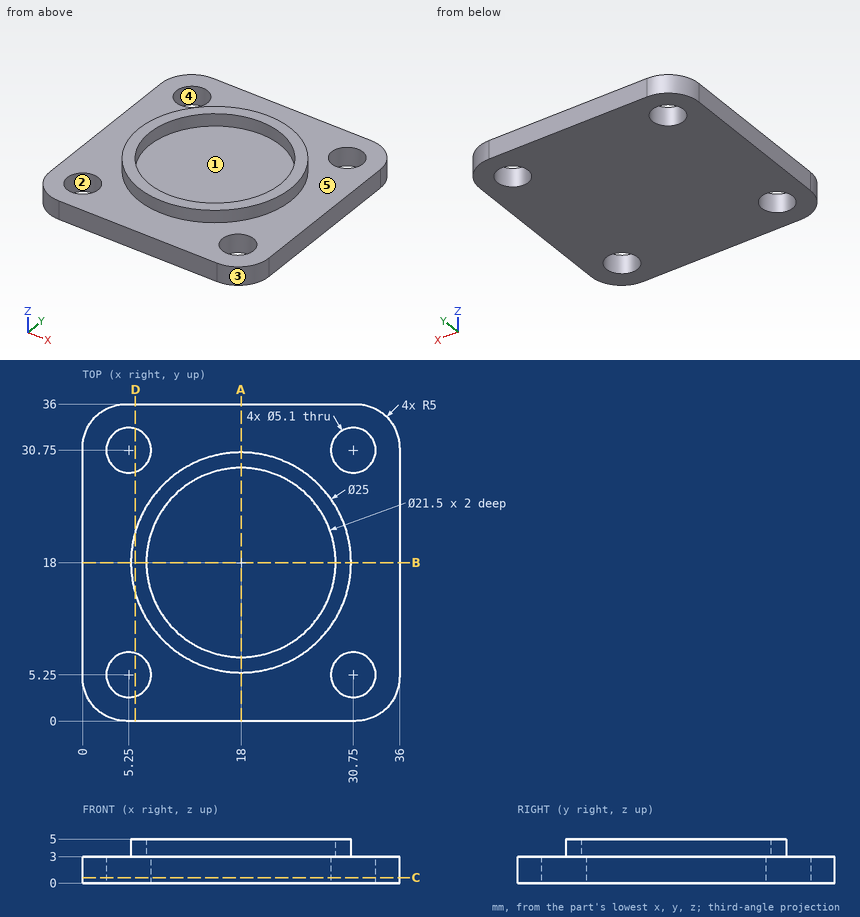
The figure shows three views and two pictorial views of one solid part (mm, origin at its lowest corner). Answer the questions. A direction names the side the tool comes from. Round coordinates to 2 decimals unless told otherwise and drop trailing zeros. Loops run counter-clockwise (first coordinate to the right, second up) from the corner with the lowest first, then second, coordinate; pieces in that order, holes last. Notation, with made-up numbers: (39, 44.25) - (81, 44.25) arc R22 cw to (81, 50.25) - close; hole circle Ø8 at (52, -30). An arc over 180 degrees is marked (long way). One line per question, with ' | ' between items. Start each with the question number.
Q1. Flat-ended cylindrical pins translate along their axes: pin 1 (6 mm diameter, centred on x = 30.75, y = 5.25, fed in from +Z); pin 2 (1 mm diameter, centred on x = 26.5, z = 4, fed in from +Y); pin 3 (3 mm diameter, centred on x = 5.25, y = 30.75, fed in from +Z). Find the tip coordinate at first contact, or state that the pin passes through.
Q2. For a pull along X with two mould halves and no side action, classify the marked faces 3, 4 and 5 as +X half, -X half, draft (parallel to the pull), parting line (faces both ways), or undercut.
Q3. Section C-C on z = 0.6 is taken. Give the vertices of the cut face in (x, y).
Q4. Section D-D on x = 6 is taken. Give the vertices of the cut face in (y, z), plus the area to 3 significant figures.
Q5. Find the intervals of material crossed by L1, parallel to Y at x = 30.75, z = 2.2; L2, parallel to Y at x = 18, z = 3.8; L3, parallel to X at y = 4.5, z = 2.2, in increasing order.
Q6. Section A-A on x = 18 is taken. Give the vertices of the cut face in (y, z).
Q7. For the marked faces 1 and 2, determine the directions among +Z, -Z, +X, -X, +Y, -Y from which every point of the face is accessible in a straight line to the end or side of a thin tool.
Established:
1) pin 1: z = 3 | pin 2: y = 27.6 | pin 3: through
2) face 3: +X half | face 4: undercut | face 5: draft
3) outline: (0, 5) arc R5 ccw to (5, 0) - (31, 0) arc R5 ccw to (36, 5) - (36, 31) arc R5 ccw to (31, 36) - (5, 36) arc R5 ccw to (0, 31) - close; hole circle Ø5.1 at (5.25, 5.25); hole circle Ø5.1 at (5.25, 30.75); hole circle Ø5.1 at (30.75, 5.25); hole circle Ø5.1 at (30.75, 30.75)
4) outline: (0, 0) - (2.81, 0) - (2.81, 3) - (0, 3) - close; (7.69, 0) - (28.31, 0) - (28.31, 3) - (21.5, 3) - (21.5, 5) - (14.5, 5) - (14.5, 3) - (7.69, 3) - close; (33.19, 0) - (36, 0) - (36, 3) - (33.19, 3) - close | area: 92.8 mm²
5) L1: 0 to 2.7, 7.8 to 28.2, 33.3 to 36 | L2: 5.5 to 7.25, 28.75 to 30.5 | L3: 0.03 to 2.81, 7.69 to 28.31, 33.19 to 35.97
6) outline: (0, 0) - (36, 0) - (36, 3) - (30.5, 3) - (30.5, 5) - (28.75, 5) - (28.75, 3) - (7.25, 3) - (7.25, 5) - (5.5, 5) - (5.5, 3) - (0, 3) - close
7) face 1: +Z | face 2: +Z, -Z
